Could you check a few things on this model? Use its own coordinates, in mm. A direction names the side the tool comes from. Give positions to 0.01 mm unless a question says otherwise; leave off trailing zeros. Loops run counter-clockwise (first coordinate to the right, second up) from the corner with the lowest first, then second, coordinate; pieces in that order, holes last. Notation, with made-up numbers: (87.5, -39) -> (146.5, -39) arc R32 ccw to (146.5, -7) -> close; hole circle Ø1 at (-38, 8.5). An arc over 180 degrees is marked (long way). Put each result on its own line as item: value.
```python
from build123d import *

# Parameters (mm, degrees)
BOSS_EXTRUDE1_DEPTH = 50.8
SKETCH2_R           = 2.4892
CUT_EXTRUDE1_DEPTH  = 76.201267443
SKETCH3_R           = 2.4892
CUT_EXTRUDE2_DEPTH  = 75.121121315


with BuildPart() as part:
    # Sketch1 → Boss-Extrude1 (new body)
    with BuildSketch(Plane(origin=(0, 0, 0), x_dir=(1, 0, 0), z_dir=(0, 1, 0))):
        Polygon((0, 0), (0, 50.8), (3.175, 50.8), (3.175, 3.175), (25.4, 3.175), (25.4, 0), align=None)
    extrude(amount=BOSS_EXTRUDE1_DEPTH)

    # Sketch2 → Cut-Extrude1 (cut, through all)
    with BuildSketch(Plane(origin=(3.175, 0, 0), x_dir=(0, 0, -1), z_dir=(1, 0, 0))):
        with Locations((38.1, 38.1)):
            Circle(SKETCH2_R)
        with Locations((38.1, 12.7)):
            Circle(SKETCH2_R)
        with Locations((12.7, 12.7)):
            Circle(SKETCH2_R)
        with Locations((12.7, 38.1)):
            Circle(SKETCH2_R)
    extrude(amount=-CUT_EXTRUDE1_DEPTH, mode=Mode.SUBTRACT)

    # Sketch3 → Cut-Extrude2 (cut, through all)
    with BuildSketch(Plane(origin=(0, 0, -3.175), x_dir=(-1, 0, 0), z_dir=(0, 0, -1))):
        with Locations((-12.7, 38.1)):
            Circle(SKETCH3_R)
        with Locations((-12.7, 12.7)):
            Circle(SKETCH3_R)
    extrude(amount=-CUT_EXTRUDE2_DEPTH, mode=Mode.SUBTRACT)


solid = part.part
```
1. For faces 1 (the face through (14, 25, -3.175)), 2 (the face through (13, 25, 0)), which set-ups out of +Z, -Z, +X, -X, +Y, -Y let a thin tool reach every point of the face, with its end or its side?
Recorded:
face 1: -Z, +X, +Y, -Y
face 2: +Z, +X, -X, +Y, -Y
2. If we section it at C-C (y = 38.1): List the corners of the cut face in (x, z) for me (3 decimals), then the cut area to 3 significant figures.
Recorded:
outline: (0, -50.8) -> (3.175, -50.8) -> (3.175, -40.589) -> (0, -40.589) -> close; (0, -35.611) -> (3.175, -35.611) -> (3.175, -15.189) -> (0, -15.189) -> close; (0, -10.211) -> (3.175, -10.211) -> (3.175, -3.175) -> (10.211, -3.175) -> (10.211, 0) -> (0, 0) -> close; (15.189, -3.175) -> (25.4, -3.175) -> (25.4, 0) -> (15.189, 0) -> close
area: 184 mm^2
3. If we section it at A-A (x = 12.7): List the corners of the cut face in (y, z) for me (3 decimals), then the cut area to 3 significant figures.
Recorded:
outline: (0, -3.175) -> (10.211, -3.175) -> (10.211, 0) -> (0, 0) -> close; (15.189, -3.175) -> (35.611, -3.175) -> (35.611, 0) -> (15.189, 0) -> close; (40.589, -3.175) -> (50.8, -3.175) -> (50.8, 0) -> (40.589, 0) -> close
area: 130 mm^2
4. Thinking about a two-plate mould opening in Y: for faces 3 (the face through (0, 25, -25)), 4 (the face through (1.61, 36.59, -36.12)), 5 (the face through (2, 50.8, -16)), 6 (the face through (1.61, 15.17, -12.38)), which applies, pulls with the +Y half, pulls with the -Y half, needs draft (parallel to the pull), parting line crosses it, or undercut?
Recorded:
face 3: needs draft
face 4: undercut
face 5: pulls with the +Y half
face 6: undercut
5. I need wall thicknesses on line 1 (Z direction, x = 24.5, y = 43) (3 decimals); line 2 (X direction, y = 11, z = -31) (3 decimals). Which ranges of each line are inside material? Lowest first, please.
Recorded:
line 1: z = -3.175 to 0
line 2: x = 0 to 3.175
6. I'm going to push flat-ended pins straight in: pin 1 (1.5 mm diameter, centred on x = 6.5, y = 24, fed in from -Z) (3 decimals); pin 2 (14.5 mm diameter, centred on y = 37, z = -21.5, fed in from +X) (3 decimals). Where does each tip first touch, or does it pass through?
Recorded:
pin 1: stops at z = -3.175
pin 2: stops at x = 3.175
7. If we section it at D-D (y = 47.5): List the corners of the cut face in (x, z) for me (3 decimals), then the cut area to 3 significant figures.
Recorded:
outline: (0, -50.8) -> (3.175, -50.8) -> (3.175, -3.175) -> (25.4, -3.175) -> (25.4, 0) -> (0, 0) -> close
area: 232 mm^2
8. If we section it at B-B (z = -12.7): List the corners of the cut face in (x, y) for me (3 decimals).
Recorded:
outline: (0, 0) -> (3.175, 0) -> (3.175, 10.211) -> (0, 10.211) -> close; (0, 15.189) -> (3.175, 15.189) -> (3.175, 35.611) -> (0, 35.611) -> close; (0, 40.589) -> (3.175, 40.589) -> (3.175, 50.8) -> (0, 50.8) -> close
